The figure shows three views and two pictorial views of one solid part (mm, origin at its lowest corner). Answer the questions. Give positions to 0.01 mm unless a question says otherwise; leave off trailing zeros. Loops run counter-clockwise (first coordinate to the right, second up) from the corner with the lowest first, then second, coordinate; pieces in that order, holes last. Notation, with made-up numbers: M 84,-31.75 L 88,-31.75 A11 ccw 88,-16.75 Z; hole C 46,40 d3. An arc over 180 degrees is marked long. Answer in a Markdown table with one row per item. Add a question column.
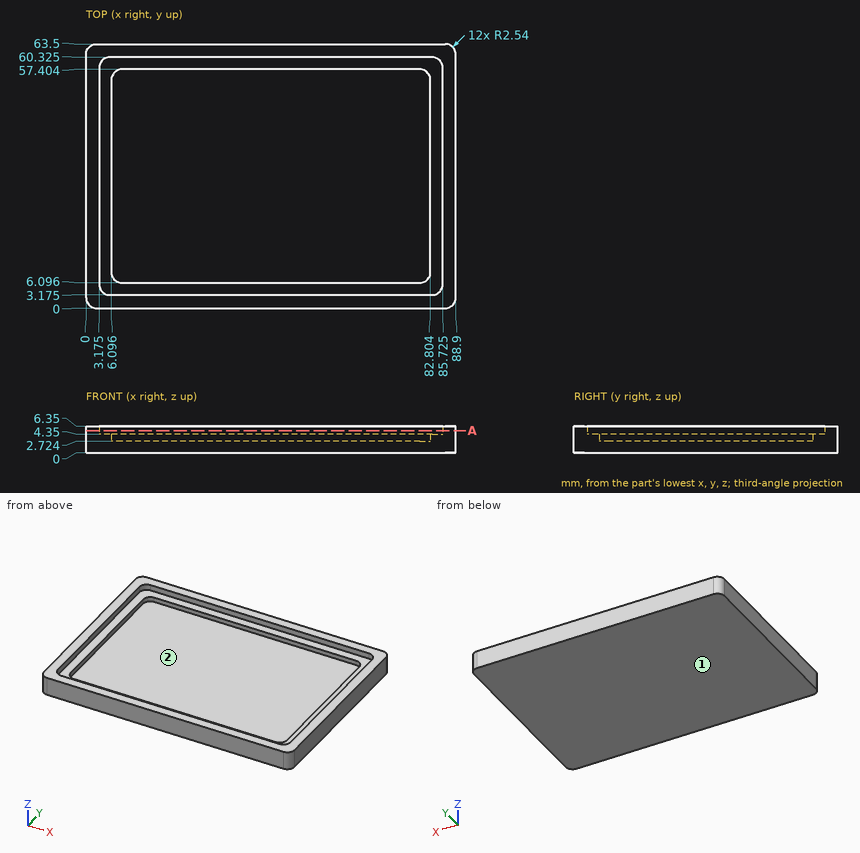
(1) Consider line 1 along X through (y, z) = (50, 3.5); line 2 along Y through (x, z) = (10.5, 5.75) (1 decimal); line 3 along Y through (x, z) = (28, 3.25). Determine where each line is inside the solid, lowest interval first. Write a range as from..to.
(2) This flat-tipped pin is pushed along its axis until it touches: P1, Ø15.5, axis at x = 51, y = 29, coming from the +Z side. Where does it stop, or does it pass through?
(3) Section A-A, the plane z = 5.25 is taken. Determine the outline of the cut face in (x, y) (1 decimal).
(4) The mould has two halves that part along Y. Classify the marked faces 1 and 2: pulls with the +Y half, pulls with the -Y half, needs draft (parallel to the pull), parting line crosses it, or undercut.
Numbers:
| question | item | result |
|---|---|---|
| 1 | line 1 | x = 0..6.1, 82.8..88.9 |
| 1 | line 2 | y = 0..3.2, 60.3..63.5 |
| 1 | line 3 | y = 0..6.1, 57.4..63.5 |
| 2 | P1 | stops at z = 2.72 |
| 3 | outline | M 0,2.5 A2.5 ccw 2.5,0 L 86.4,0 A2.5 ccw 88.9,2.5 L 88.9,61 A2.5 ccw 86.4,63.5 L 2.5,63.5 A2.5 ccw 0,61 Z; hole M 3.2,5.7 A2.5 ccw 5.7,3.2 L 83.2,3.2 A2.5 ccw 85.7,5.7 L 85.7,57.8 A2.5 ccw 83.2,60.3 L 5.7,60.3 A2.5 ccw 3.2,57.8 Z |
| 4 | face 1 | needs draft |
| 4 | face 2 | undercut |
